from build123d import *

# Parameters (mm, degrees)
CROQUIS1_R              = 1.7
SALIENTE_EXTRUIR1_DEPTH = 2
CROQUIS5_R              = 1.7
SALIENTE_EXTRUIR3_DEPTH = 1


with BuildPart() as part:
    # Croquis1 → Saliente-Extruir1 (new body)
    with BuildSketch(Plane(origin=(0, 0, 0), x_dir=(1, 0, 0), z_dir=(0, 1, 0))):
        with BuildLine():
            Line((-8, 6), (8, 6))
            Line((8, 6), (8, 3.665719575))
            ThreePointArc((8, 3.665719575), (8.133788189, 2.858848044), (8.520833333, 2.138336419))
            ThreePointArc((8.520833333, 2.138336419), (9.25, 0), (8.520833333, -2.138336419))
            ThreePointArc((8.520833333, -2.138336419), (8.133788189, -2.858848044), (8, -3.665719575))
            Line((8, -3.665719575), (8, -6))
            Line((8, -6), (-8, -6))
            Line((-8, -6), (-8, -3.665719575))
            ThreePointArc((-8, -3.665719575), (-8.133788189, -2.858848044), (-8.520833333, -2.138336419))
            ThreePointArc((-8.520833333, -2.138336419), (-9.25, 0), (-8.520833333, 2.138336419))
            ThreePointArc((-8.520833333, 2.138336419), (-8.133788189, 2.858848044), (-8, 3.665719575))
            Line((-8, 3.665719575), (-8, 6))
        make_face()
        with Locations((5.75, 0)):
            Circle(CROQUIS1_R, mode=Mode.SUBTRACT)
        with Locations((-5.75, 0)):
            Circle(CROQUIS1_R, mode=Mode.SUBTRACT)
    extrude(amount=SALIENTE_EXTRUIR1_DEPTH)

    # Croquis5 → Saliente-Extruir3 (add)
    with BuildSketch(Plane(origin=(0, 2, 0), x_dir=(1, 0, 0), z_dir=(0, 1, 0))):
        with BuildLine():
            Line((3.5, -6), (3.5, 6))
            Line((3.5, 6), (8, 6))
            Line((8, 6), (8, 3.665719575))
            ThreePointArc((8, 3.665719575), (8.133788189, 2.858848044), (8.520833333, 2.138336419))
            ThreePointArc((8.520833333, 2.138336419), (9.25, 0), (8.520833333, -2.138336419))
            ThreePointArc((8.520833333, -2.138336419), (8.133788189, -2.858848044), (8, -3.665719575))
            Line((8, -3.665719575), (8, -6))
            Line((8, -6), (3.5, -6))
        make_face()
        with Locations((5.75, 0)):
            Circle(CROQUIS5_R, mode=Mode.SUBTRACT)
    saliente_extruir3 = extrude(amount=SALIENTE_EXTRUIR3_DEPTH)

    # Simetría1: Saliente-Extruir3 across plane
    add(saliente_extruir3.mirror(Plane(origin=(0, 0, 0), x_dir=(0, 0, 1), z_dir=(1, 0, 0))))


solid = part.part
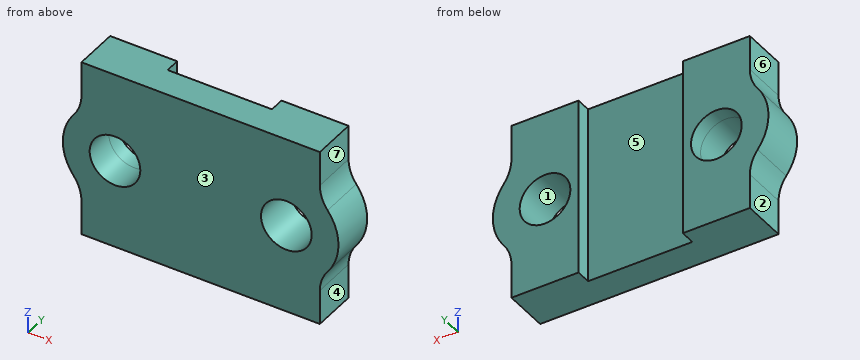
The listing builds one solid part. Answer for the finished solid, in the listing's coordinates (mm). Face numbers are marked on the shaded views. A direction names the side the tool comes from. Coordinates: 2 decimals unless noted, no trailing zeros. Loops run counter-clockwise (first coordinate to the right, second up) from the corner with the lowest first, then second, coordinate; pieces in that order, holes last. Notation, with made-up numbers: (39.5, -0.5) -> (92.5, -0.5) arc R14 cw to (92.5, 3.5) -> close; hole circle Ø4 at (56, 55.5). An arc over 180 degrees is marked (long way). Write item = value, one per line. Start each with the question number.
1) The mould has two halves that part along X. Classify the marked faces 1, 2 and 3: released by +X, released by -X, zero draft, split by the parting line, or undercut.
2) A cutting plane is placed at D-D (y = 1.05). Give the vertices of the cut face in (x, z), then the cut area to 3 significant figures.
3) Given pin 1 Ø1.2 at (y, z) = (1.5, 4.5) entering from -X; pin 2 Ø0.7 at (y, z) = (1.5, 5) entering from +X; pin 3 Ø0.5 at (y, z) = (2.5, -1) entering from -X; pin 4 Ø2 at (x, z) = (5.75, 0) entering from +Y, each flat-ended and moving along its own axis, determine where each tip first touches the part or whether it passes through.
4) A cutting plane is placed at A-A (y = 2.25). Give the vertices of the cut face in (x, z).
5) A cutting plane is placed at C-C (x = 5.75). Give the vertices of the cut face in (y, z), then the cut area to 3 significant figures.
6) A tool of negligible diameter and unlimited length cuts with its end or side. For the marked faces 4, 5, 6 and 7, from which of +Z, -Z, +X, -X, +Y, -Y can it reach the whole face along a straight path? Write none if from no direction.
7) A cutting plane is placed at B-B (z = 0). Give the vertices of the cut face in (x, y), then the cut area to 3 significant figures.
8) Straight lines are drawn through the part: line 1 (X direction, y = 2.35, z = 0); line 2 (X direction, y = 1.2, z = 0); line 3 (X direction, y = 0.55, z = -0.75). For each, find the intervals that lie inside material, in ascending order. Write a range as from..to.
Responses:
q1.face_1 = undercut
q1.face_2 = released by -X
q1.face_3 = zero draft
q2.outline = (-8.52, -2.14) arc R2.5 cw to (-8, -3.67) -> (-8, -6) -> (8, -6) -> (8, -3.67) arc R2.5 cw to (8.52, -2.14) arc R3.5 ccw to (8.52, 2.14) arc R2.5 cw to (8, 3.67) -> (8, 6) -> (-8, 6) -> (-8, 3.67) arc R2.5 cw to (-8.52, 2.14) arc R3.5 ccw to start; hole circle Ø3.4 at (-5.75, 0); hole circle Ø3.4 at (5.75, 0)
q2.area = 184 mm²
q3.pin_1 = -8
q3.pin_2 = 8
q3.pin_3 = -9.17
q3.pin_4 = through
q4.outline = (-8.52, -2.14) arc R2.5 cw to (-8, -3.67) -> (-8, -6) -> (-3.5, -6) -> (-3.5, 6) -> (-8, 6) -> (-8, 3.67) arc R2.5 cw to (-8.52, 2.14) arc R3.5 ccw to start; (3.5, -6) -> (8, -6) -> (8, -3.67) arc R2.5 cw to (8.52, -2.14) arc R3.5 ccw to (8.52, 2.14) arc R2.5 cw to (8, 3.67) -> (8, 6) -> (3.5, 6) -> close; hole circle Ø3.4 at (-5.75, 0); hole circle Ø3.4 at (5.75, 0)
q5.outline = (0, -6) -> (3, -6) -> (3, -1.7) -> (0, -1.7) -> close; (0, 1.7) -> (3, 1.7) -> (3, 6) -> (0, 6) -> close
q5.area = 25.8 mm²
q6.face_4 = -Z, +X, +Y, -Y
q6.face_5 = +Z, -Z, +Y
q6.face_6 = +Z, -X, +Y, -Y
q6.face_7 = +Z, +X, +Y, -Y
q7.outline = (-9.25, 0) -> (-7.45, 0) -> (-7.45, 3) -> (-9.25, 3) -> close; (-4.05, 0) -> (4.05, 0) -> (4.05, 3) -> (3.5, 3) -> (3.5, 2) -> (-3.5, 2) -> (-3.5, 3) -> (-4.05, 3) -> close; (7.45, 0) -> (9.25, 0) -> (9.25, 3) -> (7.45, 3) -> close
q7.area = 28.1 mm²
q8.line_1 = -9.25..-7.45, -4.05..-3.5, 3.5..4.05, 7.45..9.25
q8.line_2 = -9.25..-7.45, -4.05..4.05, 7.45..9.25
q8.line_3 = -9.17..-7.28, -4.22..4.22, 7.28..9.17
